Design review of the part built by this model. Coordinates are the model's own, in mm. Face numbers are marked on the shaded views. A direction names the side the tool comes from. Coordinates: 2 decimals unless noted, no trailing zeros. Loops run counter-clockwise (first coordinate to the right, second up) from the corner with the lowest first, then second, coordinate; pieces in that order, holes last. Notation, with made-up numbers: (-29, 6) -> (-4, 6) arc R12 ccw to (-4, 24) -> close; hole circle Ø9 at (-24, 7.5). An arc over 180 degrees is marked (long way). Answer as a JSON object with one key per item and string values.
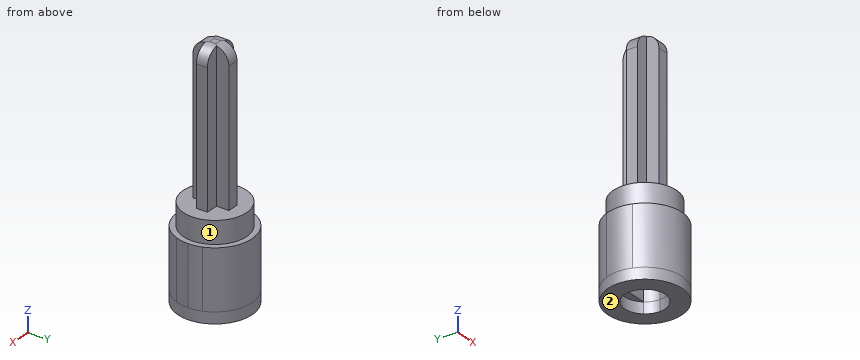
```python
from build123d import *
from build123d import SkipClean  # not in build123d's __all__

# Parameters (mm, degrees)
F1_DEPTH    = 8
F2_R        = 4.25
F3_DEPTH    = 3
F4_W        = 1.675
F4_H        = 1.5
F4_W_2      = 1.5
F4_H_2      = 1.675
F5_DEPTH    = 20
F6_T1_DEPTH = 11.5
F6_T3_DEPTH = 11.5
F7_R        = 5
F8_DEPTH    = 1.5


# Not quite as in the source:
# - a fillet or chamfer that OpenCascade refuses, or shapes differently, is made with other operations: its cross-section is extruded or revolved along the edge and cut away or added


with BuildPart() as f1:
    # F0 (on Top) → F1 (new body)
    with BuildSketch(Plane.XY):
        with BuildLine():
            ThreePointArc((4.6837484988, -1.75), (4.9203019467, -0.8891730726), (5, 0))
            ThreePointArc((5, 0), (4.9203019467, 0.8891730726), (4.6837484988, 1.75))
            Line((4.6837484988, 1.75), (2.1213203436, 1.75))
            ThreePointArc((2.1213203436, 1.75), (2.5880621075, 0.9297497123), (2.75, 0))
            ThreePointArc((2.75, 0), (2.5880621075, -0.9297497123), (2.1213203436, -1.75))
            Line((2.1213203436, -1.75), (4.6837484988, -1.75))
        make_face()
        with BuildLine():
            Line((2.1213203436, 1.75), (4.6837484988, 1.75))
            ThreePointArc((4.6837484988, 1.75), (0, 5), (-4.6837484988, 1.75))
            Line((-4.6837484988, 1.75), (-2.1213203436, 1.75))
            ThreePointArc((-2.1213203436, 1.75), (0, 2.75), (2.1213203436, 1.75))
        make_face()
        with BuildLine():
            ThreePointArc((-4.6837484988, -1.75), (0, -5), (4.6837484988, -1.75))
            Line((4.6837484988, -1.75), (2.1213203436, -1.75))
            ThreePointArc((2.1213203436, -1.75), (0, -2.75), (-2.1213203436, -1.75))
            Line((-2.1213203436, -1.75), (-4.6837484988, -1.75))
        make_face()
        with BuildLine():
            Line((-2.1213203436, 1.75), (-4.6837484988, 1.75))
            ThreePointArc((-4.6837484988, 1.75), (-5, 0), (-4.6837484988, -1.75))
            Line((-4.6837484988, -1.75), (-2.1213203436, -1.75))
            ThreePointArc((-2.1213203436, -1.75), (-2.75, 0), (-2.1213203436, 1.75))
        make_face()
        with BuildLine():
            Line((-2.1213203436, 1.75), (2.1213203436, 1.75))
            ThreePointArc((2.1213203436, 1.75), (0, 2.75), (-2.1213203436, 1.75))
        make_face()
        with BuildLine():
            ThreePointArc((-2.1213203436, -1.75), (0, -2.75), (2.1213203436, -1.75))
            Line((2.1213203436, -1.75), (-2.1213203436, -1.75))
        make_face()
    extrude(amount=F1_DEPTH)

    # F2 (on face) → F3 (join)
    with BuildSketch(Plane.XY.offset(8)):
        Circle(F2_R)
    extrude(amount=F3_DEPTH)

    # F4 (on face) → F5 (join)
    with BuildSketch(Plane.XY.offset(11)):
        with Locations((-1.5875, 0)):
            Rectangle(F4_W, F4_H)
        Rectangle(F4_W_2, F4_H)
        with Locations((0, 1.5875)):
            Rectangle(F4_W_2, F4_H_2)
        with Locations((1.5875, 0)):
            Rectangle(F4_W, F4_H)
        with Locations((0, -1.5875)):
            Rectangle(F4_W_2, F4_H_2)
    extrude(amount=F5_DEPTH)

    # F6: fillet of radius 2 on 4 edges, made by hand

    # F6_s2 → F6_t1 (cut)
    with BuildSketch(Plane.YZ.offset(-5.75)):
        with BuildLine():
            ThreePointArc((2.425, 29), (1.8392135624, 30.4142135624), (0.425, 31))
            Line((0.425, 31), (2.425, 31))
            Line((2.425, 31), (2.425, 29))
        make_face()
        with BuildLine():
            ThreePointArc((-2.425, 29), (-1.8392135624, 30.4142135624), (-0.425, 31))
            Line((-0.425, 31), (-2.425, 31))
            Line((-2.425, 31), (-2.425, 29))
        make_face()
    extrude(amount=F6_T1_DEPTH, mode=Mode.SUBTRACT)

    # F6_s4 → F6_t3 (cut)
    with BuildSketch(Plane.XZ.offset(-5.75)):
        with BuildLine():
            ThreePointArc((2.425, 29), (1.8392135624, 30.4142135624), (0.425, 31))
            Line((0.425, 31), (2.425, 31))
            Line((2.425, 31), (2.425, 29))
        make_face()
        with BuildLine():
            ThreePointArc((-2.425, 29), (-1.8392135624, 30.4142135624), (-0.425, 31))
            Line((-0.425, 31), (-2.425, 31))
            Line((-2.425, 31), (-2.425, 29))
        make_face()
    extrude(amount=F6_T3_DEPTH, mode=Mode.SUBTRACT)

    # F7 (on face) → F8 (join)
    with BuildSketch(Plane(origin=(0, 0, 0), x_dir=(1, 0, 0), z_dir=(0, 0, -1))):
        Circle(F7_R)
        with BuildLine():
            ThreePointArc((2.1213203436, 1.75), (2.5880621075, 0.9297497123), (2.75, 0))
            ThreePointArc((2.75, 0), (2.5880621075, -0.9297497123), (2.1213203436, -1.75))
            ThreePointArc((2.1213203436, -1.75), (0, -2.75), (-2.1213203436, -1.75))
            ThreePointArc((-2.1213203436, -1.75), (-2.75, 0), (-2.1213203436, 1.75))
            ThreePointArc((-2.1213203436, 1.75), (0, 2.75), (2.1213203436, 1.75))
        make_face(mode=Mode.SUBTRACT)
    with SkipClean():  # cleaning this boolean's faces spoils the solid; the shape is the same uncleaned
        extrude(amount=F8_DEPTH)


solid = f1.part
```
1) Clearance check with flat-ended pins moving along their axes: pin 1 Ø0.5 at (x, z) = (-1.5, 25.5) entering from -Y; pin 2 Ø1.3 at (y, z) = (-1.5, 18.5) entering from +X; pin 3 Ø1.1 at (x, y) = (0, -2) entering from -Z. State where each tip first meets the part, or that it passes through.
Completed:
{"pin 1": "y = -0.75", "pin 2": "x = 0.75", "pin 3": "z = 0"}
2) Add section A-A, the plane z = 6.5. Give the boundary of the cut face in (x, y), and give its area (3 significant figures).
Completed:
{"outline": "circle Ø10 at (0, 0); hole (-2.12, -1.75) -> (2.12, -1.75) arc R2.75 ccw to (2.12, 1.75) -> (-2.12, 1.75) arc R2.75 ccw to start", "area": "60.7 mm²"}
3) For the marked faces 1 and 2, list the 3-axis set-ups (+Z, -Z, +X, -X, +Y, -Y) from which the entire face can be reached by the end or side of a thin tool; tool diameter is ignored.
Completed:
{"face 1": "+Z", "face 2": "-Z, +X, -X, +Y, -Y"}
4) Add section B-B, the plane x = 0. Give the boundary of the cut face in (y, z) (3 decimals), and give its area (3 significant figures).
Completed:
{"outline": "(-5, -1.5) -> (-2.75, -1.5) -> (-2.75, 0) -> (-1.75, 0) -> (-1.75, 8) -> (1.75, 8) -> (1.75, 0) -> (2.75, 0) -> (2.75, -1.5) -> (5, -1.5) -> (5, 8) -> (4.25, 8) -> (4.25, 11) -> (2.425, 11) -> (2.425, 29) arc R2 ccw to (0.425, 31) -> (-0.425, 31) arc R2 ccw to (-2.425, 29) -> (-2.425, 11) -> (-4.25, 11) -> (-4.25, 8) -> (-5, 8) -> close", "area": "180 mm²"}
5) Wall thickness on probe 1 along Z at (x, y) = (0, -0.5); probe 2 along Y at (x, z) = (0.5, 15) (3 decimals); probe 3 along Z at (x, y) = (-3.25, -0.25): over which ranges is each line inside the solid? List them lowest first.
Completed:
{"probe 1": "8 to 31", "probe 2": "-2.425 to 2.425", "probe 3": "-1.5 to 11"}
6) Add section C-C, the plane z = 20. Give the boundary of the cut face in (x, y) (3 decimals).
Completed:
{"outline": "(-2.425, -0.75) -> (-0.75, -0.75) -> (-0.75, -2.425) -> (0.75, -2.425) -> (0.75, -0.75) -> (2.425, -0.75) -> (2.425, 0.75) -> (0.75, 0.75) -> (0.75, 2.425) -> (-0.75, 2.425) -> (-0.75, 0.75) -> (-2.425, 0.75) -> close"}
